from build123d import *

# Parameters (mm, degrees)
SKETCH1_W           = 95
SKETCH1_H           = 69
BOSS_EXTRUDE1_DEPTH = 3
SKETCH2_W           = 95
SKETCH2_H           = 3
BOSS_EXTRUDE2_DEPTH = 100
SKETCH3_W           = 95
SKETCH3_H           = 3
BOSS_EXTRUDE3_DEPTH = 100
SKETCH4_W           = 95
SKETCH4_H           = 3
CUT_EXTRUDE1_DEPTH  = 100
SKETCH5_W           = 25
SKETCH5_H           = 36
CUT_EXTRUDE2_DEPTH  = 1.5
SKETCH6_W           = 30
SKETCH6_H           = 30
CUT_EXTRUDE3_DEPTH  = 1.5
SKETCH7_R           = 1.5
CUT_EXTRUDE5_DEPTH  = 131.052204064
CUT_EXTRUDE6_DEPTH  = 131.052204064
SKETCH9_W           = 13
SKETCH9_H           = 4
CUT_EXTRUDE9_DEPTH  = 10


with BuildPart() as part:
    # Sketch1 → Boss-Extrude1 (new body)
    with BuildSketch(Plane(origin=(0, 0, 0), x_dir=(1, 0, 0), z_dir=(0, 1, 0))):
        with Locations((4.879154079, 9.171450151)):
            Rectangle(SKETCH1_W, SKETCH1_H)
    extrude(amount=-BOSS_EXTRUDE1_DEPTH)

    # Sketch2 → Boss-Extrude2 (add)
    with BuildSketch(Plane(origin=(0, 0, 0), x_dir=(1, 0, 0), z_dir=(0, 1, 0))):
        with Locations((4.879154079, -23.828549849)):
            Rectangle(SKETCH2_W, SKETCH2_H)
    extrude(amount=BOSS_EXTRUDE2_DEPTH)

    # Sketch3 → Boss-Extrude3 (add)
    with BuildSketch(Plane(origin=(0, 0, 0), x_dir=(1, 0, 0), z_dir=(0, 1, 0))):
        with Locations((4.879154079, 42.171450151)):
            Rectangle(SKETCH3_W, SKETCH3_H)
    extrude(amount=BOSS_EXTRUDE3_DEPTH)

    # Sketch4 → Cut-Extrude1 (cut)
    with BuildSketch(Plane(origin=(0, 0, -43.671450151), x_dir=(-1, 0, 0), z_dir=(0, 0, -1))):
        with Locations((-4.879154079, 98.5)):
            Rectangle(SKETCH4_W, SKETCH4_H)
    extrude(amount=-CUT_EXTRUDE1_DEPTH, mode=Mode.SUBTRACT)

    # Sketch5 → Cut-Extrude2 (cut)
    with BuildSketch(Plane(origin=(0, 0, -43.671450151), x_dir=(-1, 0, 0), z_dir=(0, 0, -1))):
        with Locations((-9.879154079, 20)):
            Rectangle(SKETCH5_W, SKETCH5_H)
    extrude(amount=-CUT_EXTRUDE2_DEPTH, mode=Mode.SUBTRACT)

    # Sketch6 → Cut-Extrude3 (cut)
    with BuildSketch(Plane.XZ.offset(3)):
        with Locations((7.379154079, -18.671450151)):
            Rectangle(SKETCH6_W, SKETCH6_H)
    extrude(amount=-CUT_EXTRUDE3_DEPTH, mode=Mode.SUBTRACT)

    # Sketch7 → Cut-Extrude5 (cut, through all)
    with BuildSketch(Plane(origin=(0, 0, -43.671450151), x_dir=(-1, 0, 0), z_dir=(0, 0, -1))):
        with Locations((34.620845921, 92)):
            Circle(SKETCH7_R)
        with Locations((-46.379154079, 92)):
            Circle(SKETCH7_R)
    extrude(amount=-CUT_EXTRUDE5_DEPTH, mode=Mode.SUBTRACT)

    # Sketch8 → Cut-Extrude6 (cut, through all)
    with BuildSketch(Plane(origin=(0, 0, -43.671450151), x_dir=(-1, 0, 0), z_dir=(0, 0, -1))):
        Polygon((42.620845921, -3), (17.620845921, -3), (42.620845921, 27), align=None)
    extrude(amount=-CUT_EXTRUDE6_DEPTH, mode=Mode.SUBTRACT)

    # Sketch9 → Cut-Extrude9 (cut)
    with BuildSketch(Plane(origin=(0, 0, -43.671450151), x_dir=(-1, 0, 0), z_dir=(0, 0, -1))):
        with Locations((-9.879154079, 84)):
            Rectangle(SKETCH9_W, SKETCH9_H)
    extrude(amount=-CUT_EXTRUDE9_DEPTH, mode=Mode.SUBTRACT)


solid = part.part
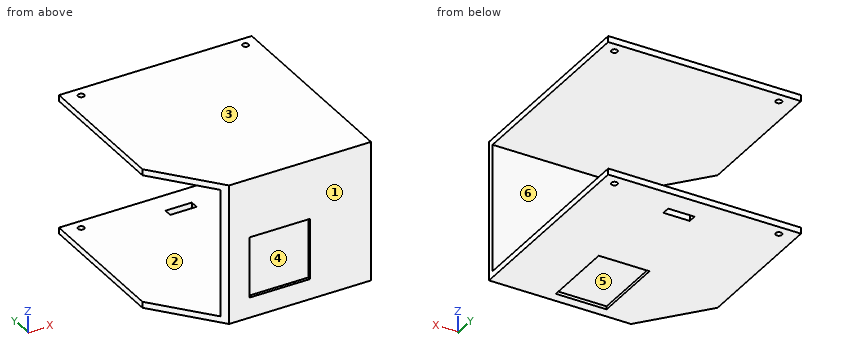
Check sheet for the modelled part. Datum: model origin and axes. Units: mm. Face numbers are marked on the shaded views. A direction names the side the tool comes from. Give positions to 0.01 mm unless a question says otherwise; leave off trailing zeros. Loops run counter-clockwise (first coordinate to the right, second up) from the corner with the lowest first, then second, coordinate; pieces in that order, holes last. Notation, with made-up numbers: M 45,60 L 97,60 A18 cw 97,86 Z; hole C 8,80 d7. An arc over 180 degrees is marked long. Answer as a JSON object with one key per item and string values. Group by question number.
Q1. Material ranges on line 1 along Z through (x, y) = (-11, 12); line 2 along Z through (x, y) = (12.5, 5); line 3 along Y through (x, z) = (-1.5, -11.5), recorded low to high. Write a range as [from, to].
Q2. Cross-section at B-B on y = 33. Record the cut outline in (x, z).
Q3. Go/stop test with flat-tipped pins: P1, Ø5, axis at x = -5, z = -29.5, coming from the +Y side; P2, Ø2.5, axis at x = 46.38, y = 92, coming from the +Z side; P3, Ø1.2, axis at y = -2.5, z = -20, coming from the -X side. Record where each tip stops, or that it passes through.
Q4. Cross-section at D-D on z = -30. Record the cut outline in (x, y).
Q5. Release check for a two-part mould opening along Y. For the marked faces 3, 4, 5 and 6 record: released by +Y, released by -Y, zero draft, split by the parting line, or undercut.
Q6. Access from +Z, -Z, +X, -X, +Y, -Y to the whole of each face (thin tool, end or side, straight path). Record for the marked faces 1 and 2.
Q7. Cross-section at C-C on x = -16. Record the cut outline in (y, z), then the cut area to 3 significant figures.
Q8. Cross-section at A-A on y = 92. Record the cut outline in (x, z), then the cut area to 3 significant figures.
Evaluation:
{
 "1": {"line 1": "z = [-43.67, -40.67], [22.33, 25.33]", "line 2": "z = [-42.17, -40.67], [22.33, 25.33]", "line 3": "y = [-1.5, 0]"},
 "2": {"outline": "M -42.62,-43.67 L -2.62,-43.67 L -2.62,-42.17 L 22.38,-42.17 L 22.38,-43.67 L 52.38,-43.67 L 52.38,-40.67 L -42.62,-40.67 Z; M -42.62,22.33 L 52.38,22.33 L 52.38,25.33 L -42.62,25.33 Z"},
 "3": {"P1": "stops at y = 0", "P2": "passes through", "P3": "stops at x = -18.54"},
 "4": {"outline": "M -20.12,0 L -17.62,-3 L -7.62,-3 L -7.62,-1.5 L 22.38,-1.5 L 22.38,-3 L 52.38,-3 L 52.38,0 Z"},
 "5": {"face 3": "zero draft", "face 4": "released by -Y", "face 5": "undercut", "face 6": "released by +Y"},
 "6": {"face 1": "+Z, -Z, +X, -X, -Y", "face 2": "+X, -X, +Y"},
 "7": {"outline": "M -3,-43.67 L 97,-43.67 L 97,-40.67 L 0,-40.67 L 0,22.33 L 97,22.33 L 97,25.33 L -3,25.33 Z", "area": "789 mm2"},
 "8": {"outline": "M -42.62,-43.67 L -36.12,-43.67 L -36.12,-40.67 L -42.62,-40.67 Z; M -42.62,22.33 L -36.12,22.33 L -36.12,25.33 L -42.62,25.33 Z; M -33.12,-43.67 L 44.88,-43.67 L 44.88,-40.67 L -33.12,-40.67 Z; M -33.12,22.33 L 44.88,22.33 L 44.88,25.33 L -33.12,25.33 Z; M 47.88,-43.67 L 52.38,-43.67 L 52.38,-40.67 L 47.88,-40.67 Z; M 47.88,22.33 L 52.38,22.33 L 52.38,25.33 L 47.88,25.33 Z", "area": "534 mm2"}
}
